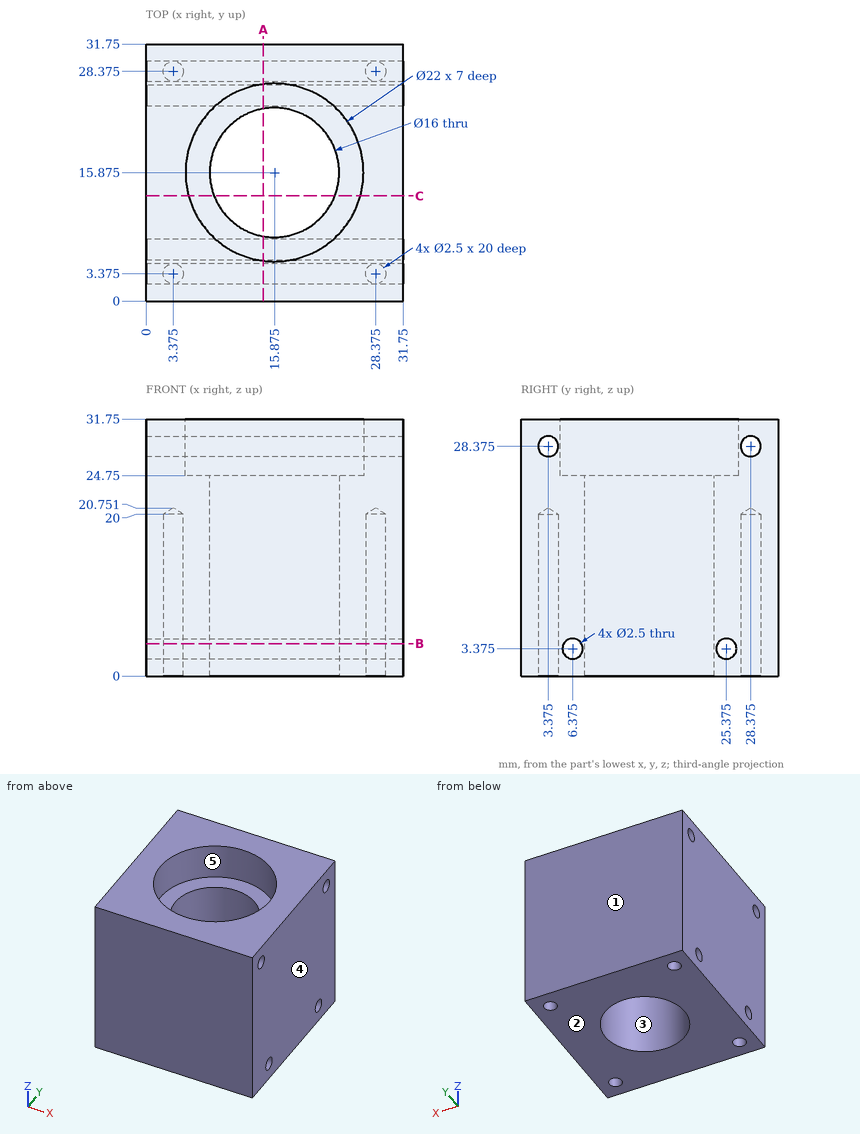
The figure shows three views and two pictorial views of one solid part (mm, origin at its lowest corner). Answer the questions. A direction names the side the tool comes from. Round coordinates to 2 decimals unless told otherwise and drop trailing zeros. Loops run counter-clockwise (first coordinate to the right, second up) from the corner with the lowest first, then second, coordinate; pieces in that order, holes last. Notation, with made-up numbers: (24, -2.5) - (45, -2.5) arc R20 cw to (45, 9.5) - close; hole circle Ø11 at (27, 35.25). An arc over 180 degrees is marked (long way). Use one line per item in the form item = value. Start each with the question number.
(1) Determine the mould class of the marked faces 1, 2 and 3 for opening direction Y: +Y half, -Y half, draft (parallel to the pull), parting line (faces both ways), or undercut.
(2) Find section A-A on x = 14.5. Determine the outline of the cut face in (y, z) (3 decimals).
(3) Find section C-C on y = 13. Determine the outline of the cut face in (x, z).
(4) Which of the six approach directions +Z, -Z, +X, -X, +Y, -Y give full straight-line access (tool end or side, diameter ignored) to the marked faces 4 and 5?
(5) Flat-ended cylindrical pins translate along their axes: P1, Ø14.5, axis at x = 15.875, y = 15.875, coming from the -Z side; P2, Ø2, axis at x = 3.375, y = 3.375, coming from the -Z side. Find the tip coordinate at first contact, or state that the pin passes through.
(6) Find section B-B on z = 4. Give the number of separate pieces and of enclosed holes in the cut face, and give its area (3 significant figures).
(7) Consider line 1 (Y direction, x = 29.5, z = 9.5); line 2 (Y direction, x = 4.5, z = 3); line 3 (Y direction, x = 3, z = 18). Determine where each line is inside the solid, lowest interval first.
Answer list:
q1.face_1 = +Y half
q1.face_2 = draft
q1.face_3 = undercut
q2.outline = (0, 0) - (7.994, 0) - (7.994, 24.75) - (4.961, 24.75) - (4.961, 31.75) - (0, 31.75) - close; (23.756, 0) - (31.75, 0) - (31.75, 31.75) - (26.789, 31.75) - (26.789, 24.75) - (23.756, 24.75) - close; hole circle Ø2.5 at (3.375, 28.375); hole circle Ø2.5 at (6.375, 3.375); hole circle Ø2.5 at (25.375, 3.375); hole circle Ø2.5 at (28.375, 28.375)
q3.outline = (0, 0) - (8.41, 0) - (8.41, 24.75) - (5.26, 24.75) - (5.26, 31.75) - (0, 31.75) - close; (23.34, 0) - (31.75, 0) - (31.75, 31.75) - (26.49, 31.75) - (26.49, 24.75) - (23.34, 24.75) - close
q4.face_4 = +Z, -Z, +X, +Y, -Y
q4.face_5 = +Z
q5.P1 = through
q5.P2 = 20.15
q6.separate_pieces = 3
q6.enclosed_holes = 5
q6.area = 650 mm^2
q7.line_1 = 0 to 2.83, 3.92 to 27.83, 28.92 to 31.75
q7.line_2 = 0 to 2.83, 3.92 to 5.18, 7.57 to 24.18, 26.57 to 27.83, 28.92 to 31.75
q7.line_3 = 0 to 2.18, 4.57 to 27.18, 29.57 to 31.75
